Here's how the part is built. I have some questions about the finished solid (model axes, mm). A direction names the side the tool comes from. Give positions to 0.01 mm unless a question says otherwise; leave off trailing zeros. Write each loop counter-clockwise with the first axis right and the second up, starting at its lowest first coordinate (ties: lowest second). Pieces come first, ordered by that corner, then holes. Notation, with made-up numbers: (-24.5, -22.75) -> (-17.5, -22.75) arc R31 cw to (-17.5, 9.25) -> close; hole circle Ø1 at (21.25, 35.5). An arc over 180 degrees is marked (long way). Use one line per item in the form item = value.
```python
from build123d import *


with BuildPart() as part:
    # Sketch1 → Revolve1 (revolve)
    with BuildSketch(Plane.XY):
        with BuildLine():
            Line((47.5, 0), (47.5, 3.25))
            ThreePointArc((47.5, 3.25), (49.696699141, 8.553300859), (55, 10.75))
            Line((55, 10.75), (55, 11.75))
            Line((55, 11.75), (53, 11.75))
            ThreePointArc((53, 11.75), (47.519922446, 9.480077554), (45.25, 4))
            Line((45.25, 4), (46.25, 4))
            Line((46.25, 4), (46.25, 0))
            Line((46.25, 0), (47.5, 0))
        make_face()
    revolve(axis=Axis((0, 0, 0), (0, 1, 0)))


solid = part.part
```
Q1. If we mould it in two halves opening along Z, with no side actions, what happens to faces 1 (the face through (-11.923, 11.257, 53.692)), 2 (the face through (24.86, 1.97, -39)), 3 (the face through (-29, 11.75, -45))? For each: +Z half, -Z half, draft (parallel to the pull), parting line (faces both ways), or undercut.
Result set:
face_1 = parting line
face_2 = undercut
face_3 = draft
Q2. I want a section at A-A, the plane z = 0. Write out the boundary of the cut face in (x, y).
Result set:
outline = (-55, 10.75) arc R7.5 cw to (-47.5, 3.25) -> (-47.5, 0) -> (-46.25, 0) -> (-46.25, 4) -> (-45.25, 4) arc R7.75 ccw to (-53, 11.75) -> (-55, 11.75) -> close; (45.25, 4) -> (46.25, 4) -> (46.25, 0) -> (47.5, 0) -> (47.5, 3.25) arc R7.5 cw to (55, 10.75) -> (55, 11.75) -> (53, 11.75) arc R7.75 ccw to start
Q3. I want a section at B-B, the plane x = 0. Write out the boundary of the cut face in (y, z), and give its area (3 significant figures).
Result set:
outline = (0, -47.5) -> (3.25, -47.5) arc R7.5 cw to (10.75, -55) -> (11.75, -55) -> (11.75, -53) arc R7.75 ccw to (4, -45.25) -> (4, -46.25) -> (0, -46.25) -> close; (0, 46.25) -> (4, 46.25) -> (4, 45.25) arc R7.75 ccw to (11.75, 53) -> (11.75, 55) -> (10.75, 55) arc R7.5 cw to (3.25, 47.5) -> (0, 47.5) -> close
area = 58.2 mm2
Q4. I want a section at C-C, the plane y = 7.25. Write out the boundary of the cut face in (x, z).
Result set:
outline = circle Ø97.31 at (0, 0); hole circle Ø91.93 at (0, 0)
Q5. If I drill on line 1 along X through (y, z) = (1.05, 0); line 2 along Z through (x, y) = (-31.5, 1.25), over which ranges is the centre line in solid material (lowest first)? Write a range as from..to.
Result set:
line_1 = -47.5..-46.25, 46.25..47.5
line_2 = -35.55..-33.86, 33.86..35.55
Q6. Will these pins go through, and if not, where does the flat tip stop? pin 1 Ø1.5 at (x, z) = (-41, -30) entering from +Y; pin 2 Ø1 at (x, y) = (-31.5, 7) entering from +Z; pin 3 Ø1 at (x, z) = (-28.5, -40) entering from -Y.
Result set:
pin_1 = 11.61
pin_2 = 37.47
pin_3 = 7.18
Q7. Which directions (+Z, -Z, +X, -X, +Y, -Y) give clear straight access to the entire face, cutting with the end or side of a thin tool? Please do faces 4 (the face through (-10, 0, 46)), 5 (the face through (-10.3, 1.65, 46.37)).
Result set:
face_4 = +Z, -Z, +X, -X, -Y
face_5 = -Y
